from build123d import *

# Parameters (mm, degrees)
ZKOSEN_1_SIZE            = 1
ODEBRAT_VYSUNUT_M1_DEPTH = 7.5
ODEBRAT_VYSUNUT_M2_DEPTH = 5.5


with BuildPart() as part:
    # Skica1 → Rotovat1 (revolve)
    with BuildSketch(Plane.XY):
        Polygon((0, 0), (0, 22.5), (15, 22.5), (15, 30), (25, 30), (25, 22.5), (115, 22.5), (115, 21.25), (117, 21.25), (117, 22.5), (185, 22.5), (185, 20), (230, 20), (230, 0), align=None)
    revolve(axis=Axis((-258.80539499, 0, 0), (1, 0, 0)))

    # Zkosení1
    zkosen_1_edges = [part.edges().sort_by_distance(p)[0] for p in [
        (185, -22.5, 0),
        (230, -20, 0),
    ]]
    chamfer(zkosen_1_edges, length=ZKOSEN_1_SIZE)

    # Skica6 → Odebrat vysunutím1 (cut)
    with BuildSketch(Plane(origin=(0, 20, 0), x_dir=(1, 0, 0), z_dir=(0, 1, 0))):
        with BuildLine():
            Line((230, -3), (190, -3))
            ThreePointArc((190, -3), (187, 0), (190, 3))
            Line((190, 3), (230, 3))
            ThreePointArc((230, 3), (233, 0), (230, -3))
        make_face()
    extrude(amount=-ODEBRAT_VYSUNUT_M1_DEPTH, mode=Mode.SUBTRACT)

    # Skica7 → Odebrat vysunutím2 (cut)
    with BuildSketch(Plane(origin=(0, 22.5, 0), x_dir=(1, 0, 0), z_dir=(0, 1, 0))):
        with BuildLine():
            Line((43.5, 7), (99.5, 7))
            ThreePointArc((99.5, 7), (106.5, 0), (99.5, -7))
            Line((99.5, -7), (43.5, -7))
            ThreePointArc((43.5, -7), (36.5, 0), (43.5, 7))
        make_face()
    extrude(amount=-ODEBRAT_VYSUNUT_M2_DEPTH, mode=Mode.SUBTRACT)


solid = part.part
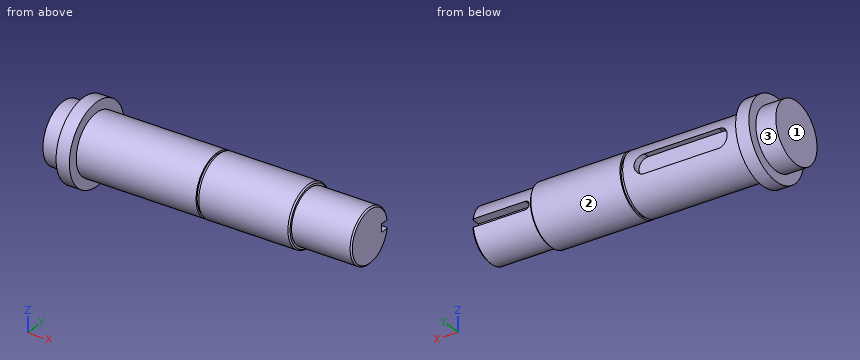
Verification items for the finished model (mm, model axes). Face numbers are marked on the shaded views. A direction names the side the tool comes from. Give positions to 0.01 mm unless a question says otherwise; leave off trailing zeros. Loops run counter-clockwise (first coordinate to the right, second up) from the corner with the lowest first, then second, coordinate; pieces in that order, holes last. Notation, with made-up numbers: (28, 63) - (84, 63) arc R38 ccw to (84, 102) - close; hole circle Ø3 at (81, 11.5). An arc over 180 degrees is marked (long way). Write item = value, one per line. Start each with the question number.
Q1. Cross-section at A-A, the plane y = 0. Enter the section's corners in (x, z).
Q2. Cross-section at D-D, the plane x = 86. Enter the section's corners in (y, z).
Q3. Tool access check on the marked faces 1, 2 and 3. Record the directions out of +Z, -Z, +X, -X, +Y, -Y that give a thin tool (end or side, any length) a straight path to the whole face; none if there is none.
Q4. Depth check by flat-ended pin: P1, Ø8, axis at x = 85.5, z = 23.5, coming from the +Y side (3 decimals); P2, Ø4, axis at x = 65, y = -5, coming from the -Z side; P3, Ø11, axis at x = 80, z = 1, coming from the +Y side. Enter the tip coordinate at first touch or a pass-through.
Q5. Cross-section at B-B, the plane x = 143. Enter the section's corners in (y, z), and give its area (3 significant figures).
Q6. Cross-section at C-C, the plane z = 26. Enter the section's corners in (x, y).
Q7. Thickness scan on line 1 (Z direction, x = 69.5, y = 6.5); line 2 (Z direction, x = 117.5, y = 12); line 3 (X direction, y = 21.5, z = -20). Record the ranges inside material, lowest first.
Answer key:
q1.outline = (0, -22.5) - (15, -22.5) - (15, -30) - (25, -30) - (25, -22.5) - (115, -22.5) - (115, -21.25) - (117, -21.25) - (117, -22.5) - (184, -22.5) - (185, -21.5) - (185, -20) - (229, -20) - (230, -19) - (230, 19) - (229, 20) - (185, 20) - (185, 21.5) - (184, 22.5) - (117, 22.5) - (117, 21.25) - (115, 21.25) - (115, 22.5) - (25, 22.5) - (25, 30) - (15, 30) - (15, 22.5) - (0, 22.5) - close
q2.outline = (17, -7) - (17, 7) - (21.38, 7) arc R22.5 ccw (long way) to (21.38, -7) - close
q3.face_1 = +Z, -Z, -X, +Y, -Y
q3.face_2 = +X
q3.face_3 = -X
q4.P1 = 11.225
q4.P2 = -22.3
q4.P3 = 17
q5.outline = circle Ø45 at (0, 0)
q5.area = 1,590 mm^2
q6.outline = (15, -14.97) - (25, -14.97) - (25, 14.97) - (15, 14.97) - close
q7.line_1 = -21.54 to 21.54
q7.line_2 = -19.03 to 19.03
q7.line_3 = 15 to 25
